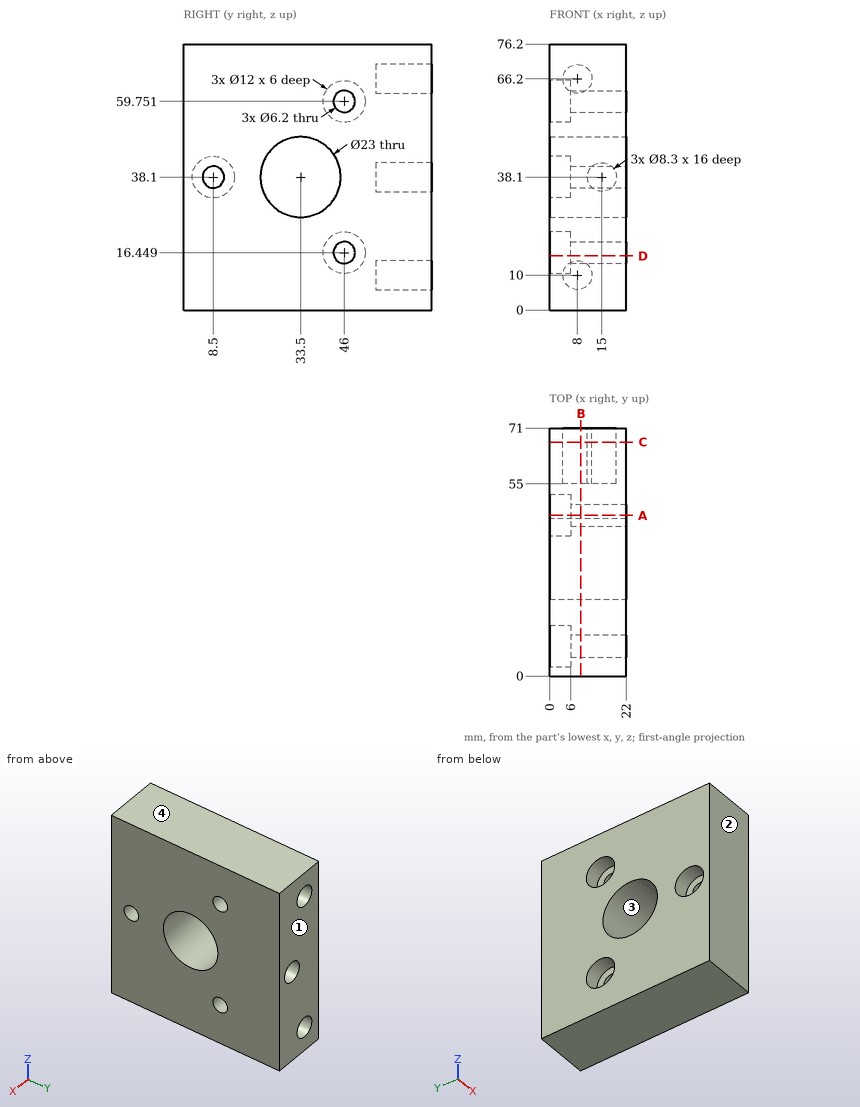
For this review, use the dimensioned drawing (mm, ordinates from the lowest corner) and the shaded views. Round coordinates to 2 decimals unless told otherwise and drop trailing zeros. Write each loop counter-clockwise with the first axis right and the second up, starting at its lowest first coordinate (ties: lowest second). Pieces come first, ordered by that corner, then holes. Notation, with made-up numbers: (83.5, 38) -> (125.5, 38) arc R16 cw to (125.5, 67) -> close; hole circle Ø1 at (-26, -7). An arc over 180 degrees is marked (long way). Use one line per item in the form item = value.
Q1. Clearance check with flat-ended pins moving along their axes: pin 1 Ø6 at (y, z) = (44.5, 17.5) entering from -X; pin 2 Ø4 at (x, z) = (16, 37) entering from +Y. State where each tip first meets the part, or that it passes through.
Resolved:
pin_1 = 6
pin_2 = 55
Q2. Consider section B-B (x = 9). State the section outline as (y, z) points, then the cut area to 3 significant figures.
Resolved:
outline = (0, 0) -> (71, 0) -> (71, 5.97) -> (55, 5.97) -> (55, 14.03) -> (71, 14.03) -> (71, 62.17) -> (55, 62.17) -> (55, 70.23) -> (71, 70.23) -> (71, 76.2) -> (0, 76.2) -> close; hole circle Ø6.2 at (8.5, 38.1); hole circle Ø23 at (33.5, 38.1); hole circle Ø6.2 at (46, 16.45); hole circle Ø6.2 at (46, 59.75)
area = 4,650 mm²
Q3. The part is to be moulded in two halves that separate along Y. For the marked faces 1, 2, 3 and 4, say which applies: released by +Y, released by -Y, zero draft, split by the parting line, or undercut.
Resolved:
face_1 = released by +Y
face_2 = released by -Y
face_3 = undercut
face_4 = zero draft
Q4. Consider section D-D (z = 15.5). State the section outline as (x, y) points (1 decimal), then the cut area to 3 significant figures.
Resolved:
outline = (0, 0) -> (22, 0) -> (22, 43) -> (6, 43) -> (6, 40.1) -> (0, 40.1) -> close; (0, 51.9) -> (6, 51.9) -> (6, 49) -> (22, 49) -> (22, 71) -> (0, 71) -> close
area = 1,400 mm²
Q5. Consider section C-C (y = 67). State the section outline as (x, z) points, then the cut area to 3 significant figures.
Resolved:
outline = (0, 0) -> (22, 0) -> (22, 76.2) -> (0, 76.2) -> close; hole circle Ø8.3 at (8, 10); hole circle Ø8.3 at (8, 66.2); hole circle Ø8.3 at (15, 38.1)
area = 1,510 mm²
Q6. Consider section A-A (y = 46). State the section outline as (x, z) points.
Resolved:
outline = (0, 0) -> (22, 0) -> (22, 13.35) -> (6, 13.35) -> (6, 10.45) -> (0, 10.45) -> close; (0, 22.45) -> (6, 22.45) -> (6, 19.55) -> (22, 19.55) -> (22, 56.65) -> (6, 56.65) -> (6, 53.75) -> (0, 53.75) -> close; (0, 65.75) -> (6, 65.75) -> (6, 62.85) -> (22, 62.85) -> (22, 76.2) -> (0, 76.2) -> close
Q7. To check wall thickness, follow probe 1 along X at (y, z) = (62, 66.2); probe 2 along Z at (x, y) = (4.15, 46); probe 3 along Z at (x, y) = (13.25, 46). State the ranges of each line that lie inside material, in increasing order. Write a range as from..to.
Resolved:
probe_1 = 0..3.85, 12.15..22
probe_2 = 0..10.45, 22.45..53.75, 65.75..76.2
probe_3 = 0..13.35, 19.55..56.65, 62.85..76.2
